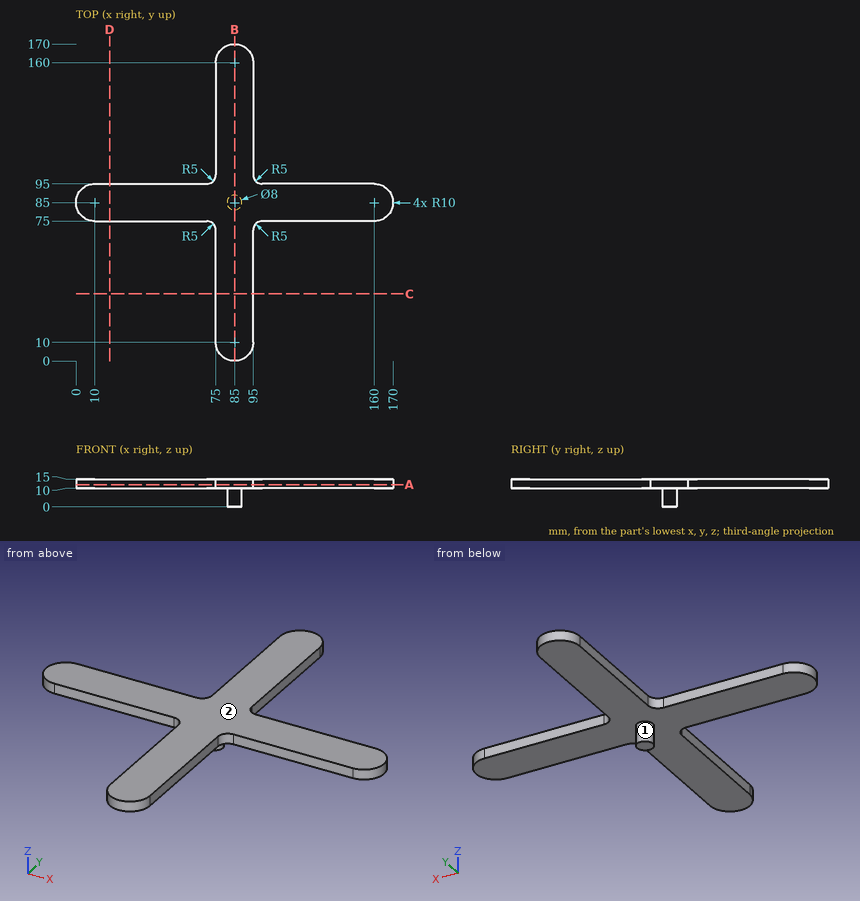
Input: dimensioned drawing with shaded views. Units: mm. Origin: part minimum x, y, z. A direction names the side the tool comes from. Coordinates: 2 decimals unless noted, no trailing zeros. Write each loop counter-clockwise with the first axis right and the second up, starting at its lowest first coordinate (ties: lowest second). Pieces come first, ordered by that corner, then holes. Notation, with made-up numbers: M 35,48.5 L 51,48.5 A14 cw 51,57.5 Z; hole C 25.25,65.25 d7. An arc over 180 degrees is marked long. Answer as a JSON object with one key per item and string values. Group by question number.
(1) Section C-C on y = 36. Output: boundary loops of the cut face in (x, z).
(2) Set-up query: the marked faces 1 and 2. Return all of +Z, -Z, +X, -X, +Y, -Y with unobstructed straight access to the full face (end or side cutting, diameter ignored); none if empty.
(3) Contact query for flat-ended pins moving along their axis: P1, Ø1, axis at y = 19, z = 12, coming from the +X side; P2, Ø4, axis at x = 130, z = 11.5, coming from the -Y side; P3, Ø5, axis at x = 88, z = 6.5, coming from the +Y side. Output: stop coordinate, or through.
(4) Ray query, line 1 along Z through (x, y) = (138, 84); line 2 along Y through (x, z) = (62, 12); line 3 along X through (y, z) = (84.5, 9.5). Return the intervals inside material, ascending. Write a range as [from, to].
(5) Section B-B on x = 85. Output: boundary loops of the cut face in (y, z), plus the area to 3 significant figures.
(6) Section A-A on z = 12. Output: boundary loops of the cut face in (x, y).
Result set:
{
 "1": {"outline": "M 75,10 L 95,10 L 95,15 L 75,15 Z"},
 "2": {"face 1": "-Z", "face 2": "+Z, +X, -X, +Y, -Y"},
 "3": {"P1": "stops at x = 95", "P2": "stops at y = 75", "P3": "stops at y = 88.97"},
 "4": {"line 1": "z = [10, 15]", "line 2": "y = [75, 95]", "line 3": "x = [81.03, 88.97]"},
 "5": {"outline": "M 0,10 L 81,10 L 81,0 L 89,0 L 89,10 L 170,10 L 170,15 L 0,15 Z", "area": "930 mm2"},
 "6": {"outline": "M 10,75 L 70,75 A5 cw 75,70 L 75,10 A10 ccw 95,10 L 95,70 A5 cw 100,75 L 160,75 A10 ccw 160,95 L 100,95 A5 cw 95,100 L 95,160 A10 ccw 75,160 L 75,100 A5 cw 70,95 L 10,95 A10 ccw Z"}
}
